Verification items for the finished model (mm, model axes). A direction names the side the tool comes from. Round coordinates to 2 decimals unless told otherwise and drop trailing zeros. Loops run counter-clockwise (first coordinate to the right, second up) from the corner with the lowest first, then second, coordinate; pieces in that order, holes last. Notation, with made-up numbers: M 34,-18 L 57,-18 A22 cw 57,-6 Z; hole C 37.5,-34 d9. An arc over 180 degrees is marked long. Answer as CSV lines item,"result".
```python
from build123d import *

# Parameters (mm, degrees)
SKETCH1_R           = 5.1
BOSS_EXTRUDE1_DEPTH = 5
SKETCH2_R           = 2.5
CUT_EXTRUDE1_DEPTH  = 35


with BuildPart() as part:
    # Sketch1 → Boss-Extrude1 (new body)
    with BuildSketch(Plane.XY):
        with BuildLine():
            Line((-84.445, 6.5), (84.445, 6.5))
            ThreePointArc((84.445, 6.5), (87.980533906, 5.035533906), (89.445, 1.5))
            Line((89.445, 1.5), (89.445, -1.5))
            ThreePointArc((89.445, -1.5), (87.980533906, -5.035533906), (84.445, -6.5))
            Line((84.445, -6.5), (-84.445, -6.5))
            ThreePointArc((-84.445, -6.5), (-87.980533906, -5.035533906), (-89.445, -1.5))
            Line((-89.445, -1.5), (-89.445, 1.5))
            ThreePointArc((-89.445, 1.5), (-87.980533906, 5.035533906), (-84.445, 6.5))
        make_face()
        Circle(SKETCH1_R, mode=Mode.SUBTRACT)
    extrude(amount=BOSS_EXTRUDE1_DEPTH)

    # Sketch2 → Cut-Extrude1 (cut)
    with BuildSketch(Plane.XY.offset(5)):
        with Locations((-81.445, 0)):
            Circle(SKETCH2_R)
        with Locations((-63.445, 0)):
            Circle(SKETCH2_R)
        with Locations(Location((63.445, 0, 0), (0, 0, 180))):
            Circle(SKETCH2_R)
        with Locations(Location((81.445, 0, 0), (0, 0, 180))):
            Circle(SKETCH2_R)
        with BuildLine():
            Line((15, 2.5), (35, 2.5))
            ThreePointArc((35, 2.5), (37.5, 0), (35, -2.5))
            Line((35, -2.5), (15, -2.5))
            ThreePointArc((15, -2.5), (12.5, 0), (15, 2.5))
        make_face()
        with BuildLine():
            Line((-15, 2.5), (-35, 2.5))
            ThreePointArc((-35, 2.5), (-37.5, 0), (-35, -2.5))
            Line((-35, -2.5), (-15, -2.5))
            ThreePointArc((-15, -2.5), (-12.5, 0), (-15, 2.5))
        make_face()
    extrude(amount=-CUT_EXTRUDE1_DEPTH, mode=Mode.SUBTRACT)


solid = part.part
```
1) Section check A-A (x = 31). Record the cut outline in (y, z).
Here are the results:
outline,"M -6.5,0 L -2.5,0 L -2.5,5 L -6.5,5 Z; M 2.5,0 L 6.5,0 L 6.5,5 L 2.5,5 Z"
2) Section check B-B (y = 0). State how many separate pieces and enclosed holes the cut face has, plus the area to 3 significant figures.
Here are the results:
separate pieces,"8"
enclosed holes,"0"
area,"493 mm^2"
3) Set-up check for faces 1 (the cylindrical face through (-12.5, -0.1, 2.5)), 2 (the flat face through (89.445, 0, 2)): record each of +Z, -Z, +X, -X, +Y, -Y from which the full face is reachable in a straight line by a thin tool's end or side.
Here are the results:
face 1,"+Z, -Z"
face 2,"+Z, -Z, +X, +Y, -Y"
4) Material ranges on probe 1 along Y at (x, z) = (-26, 2.85); probe 2 along Y at (x, z) = (-3.5, 2.05); probe 3 along X at (y, z) = (3.5, 0.95), recorded low to high.
Here are the results:
probe 1,"y = -6.5 to -2.5, 2.5 to 6.5"
probe 2,"y = -6.5 to -3.71, 3.71 to 6.5"
probe 3,"x = -89.03 to -3.71, 3.71 to 89.03"
5) Draft check along X on faces 3 (the flat face through (-89.445, 0, 2)), 4 (the cylindrical face through (-37.5, 0.1, 2.5)), 5 (the cylindrical face through (87.941, 5.074, 2.465)). Enter one of: +X half, -X half, draft (parallel to the pull), parting line (faces both ways), or undercut.
Here are the results:
face 3,"-X half"
face 4,"undercut"
face 5,"+X half"
6) Go/stop test with flat-tipped pins: pin 1 (4 mm diameter, centred on x = -81.445, y = 0, fed in from +Z); pin 2 (1.5 mm diameter, centred on y = 3.5, z = 4.5, fed in from -X). Record where each tip stops, or that it passes through.
Here are the results:
pin 1,"passes through"
pin 2,"stops at x = -89.29"
7) Section check D-D (x = 0). Record the cut outline in (y, z).
Here are the results:
outline,"M -6.5,0 L -5.1,0 L -5.1,5 L -6.5,5 Z; M 5.1,0 L 6.5,0 L 6.5,5 L 5.1,5 Z"
8) Section check C-C (z = 3.1). Record the cut outline in (x, y) (3 decimals).
Here are the results:
outline,"M -89.445,-1.5 A5 ccw -84.445,-6.5 L 84.445,-6.5 A5 ccw 89.445,-1.5 L 89.445,1.5 A5 ccw 84.445,6.5 L -84.445,6.5 A5 ccw -89.445,1.5 Z; hole C -81.445,0 d5; hole C -63.445,0 d5; hole M -35,-2.5 L -15,-2.5 A2.5 ccw -15,2.5 L -35,2.5 A2.5 ccw Z; hole C 0,0 d10.2; hole M 15,-2.5 L 35,-2.5 A2.5 ccw 35,2.5 L 15,2.5 A2.5 ccw Z; hole C 63.445,0 d5; hole C 81.445,0 d5"
